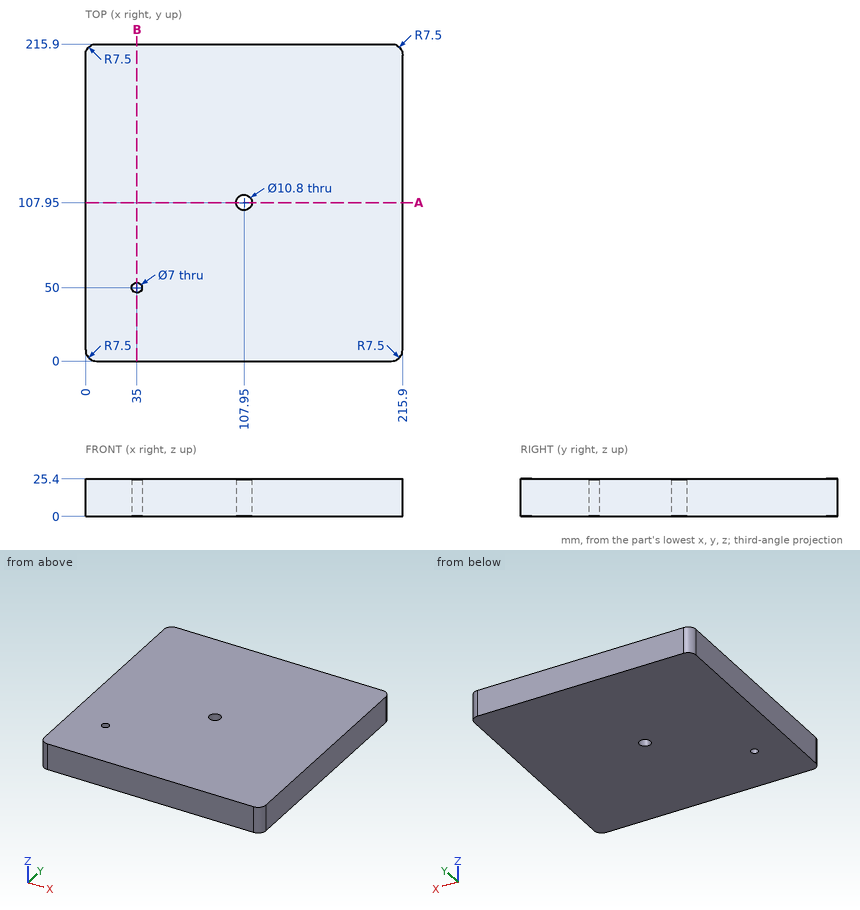
Input: dimensioned drawing with shaded views. Units: mm. Origin: part minimum x, y, z. Round coordinates to 2 decimals unless told otherwise and drop trailing zeros. Loops run counter-clockwise (first coordinate to the right, second up) from the corner with the lowest first, then second, coordinate; pieces in that order, holes last.
1) Section query A-A on y = 107.95. Return the cut outline in (x, z), plus the area to 3 significant figures.
Ans:
outline: (0, 0) - (102.55, 0) - (102.55, 25.4) - (0, 25.4) - close; (113.35, 0) - (215.9, 0) - (215.9, 25.4) - (113.35, 25.4) - close
area: 5,210 mm2
2) Section query B-B on x = 35. Return the cut outline in (y, z).
Ans:
outline: (0, 0) - (46.5, 0) - (46.5, 25.4) - (0, 25.4) - close; (53.5, 0) - (215.9, 0) - (215.9, 25.4) - (53.5, 25.4) - close
3) Material intervals for line 1 (Y direction, x = 35, z = 8); line 2 (Y direction, x = 107.95, z = 20); line 3 (X direction, y = 104, z = 8.25), sorted ascending.
Ans:
line 1: y = 0 to 46.5, 53.5 to 215.9
line 2: y = 0 to 102.55, 113.35 to 215.9
line 3: x = 0 to 104.27, 111.63 to 215.9
